Geometry: final body of the model. Coordinates: model frame, mm. Face numbers are marked on the shaded views. Round coordinates to 2 decimals unless told otherwise and drop trailing zeros. Answer as CSV lines item,"result". Start each with the question number.
Q1. Ray query, probe 1 along Z at (x, y) = (-13, -33.25); probe 2 along Y at (x, z) = (4, 5.25); probe 3 along Y at (x, z) = (-12.5, 3). Return the intervals inside material, ascending.
Q2. Mould query, pull axis X, two halves, no side actions, for the marked faces 1 and 2. Classes: pulls with the +X half, pulls with the -X half, needs draft (parallel to the pull), parting line crosses it, or undercut.
Q3. First-contact query: pin 1 (6 mm diameter, centred on y = -40.5, z = 7, fed in from -X); pin 2 (1 mm diameter, centred on y = -37, z = 2.5, fed in from +X); pin 3 (3 mm diameter, centred on y = -29, z = 6, fed in from +X); pin 4 (4 mm diameter, centred on y = -32.5, z = 6.5, fed in from +X). Flat tips, straight axial feed; report the tip coordinate or a pass-through.
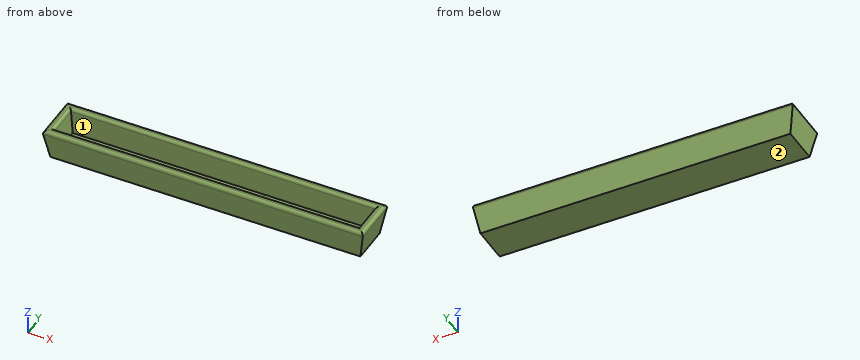
```python
from build123d import *

# Parameters (mm, degrees)
F0_W     = 100
F0_H     = 12
F1_DEPTH = 10
F1_TAPER = -10
F2_T     = -2.5
F3_R     = 1


with BuildPart() as f1:
    # F0 (on Top) → F1 (new body)
    with BuildSketch(Plane.XY):
        with Locations((-1.4750659466, -34.9569652333)):
            Rectangle(F0_W, F0_H)
    extrude(amount=F1_DEPTH, taper=F1_TAPER)

    # F2
    f2_openings = [f1.faces().sort_by_distance(p)[0] for p in [
        (-1.475066, -34.956965, 10),
    ]]
    offset(amount=F2_T, openings=f2_openings)

    # F3
    f3_edges = [f1.edges().sort_by_distance(p)[0] for p in [
        (-1.475066, -42.720235, 10),
        (-53.238336, -34.956965, 10),
        (-1.475066, -27.193695, 10),
        (50.288204, -34.956965, 10),
        (-1.475066, -29.732262, 10),
        (47.749637, -34.956965, 10),
        (-1.475066, -40.181669, 10),
        (-50.699769, -34.956965, 10),
    ]]
    fillet(f3_edges, radius=F3_R)


solid = f1.part
```
Entries:
1,probe 1,"z = 0 to 2.5"
1,probe 2,"y = -41.88 to -39.34, -30.57 to -28.03"
1,probe 3,"y = -41.49 to -38.95, -30.97 to -28.43"
2,face 1,"undercut"
2,face 2,"needs draft"
3,pin 1,"stops at x = -53.05"
3,pin 2,"stops at x = 49.05"
3,pin 3,"stops at x = 49.85"
3,pin 4,"stops at x = 50.02"
